Model file for the job. Use its own axes, mm. A direction names the side the tool comes from. Coordinates: 2 decimals unless noted, no trailing zeros. Write each loop counter-clockwise with the first axis right and the second up, starting at its lowest first coordinate (ties: lowest second). Pieces come first, ordered by that corner, then holes. Notation, with made-up numbers: (11, 78.25) -> (43, 78.25) arc R31 cw to (43, 110.25) -> close; hole circle Ø10 at (-3.75, -18). An arc over 180 degrees is marked (long way). Answer as a JSON object with one key per item and string values. Group by question number.
from build123d import *

# Parameters (mm, degrees)
F1_DEPTH  = 5.715
F2_R      = 1.143
F3_DEPTH  = 3.175
F5_R      = 4.445
F6_DEPTH  = 19.05
F4_R      = 3.175
F7_DEPTH  = 19.05
F8_R      = 4.7625
F9_DEPTH  = 6.35
F10_R     = 1.143
F11_DEPTH = 6.35
F13_DEPTH = 3.175
F14_R     = 3.175
F15_DEPTH = 0.396875


with BuildPart() as f1:
    # F0 (on Top) → F1 (new body)
    with BuildSketch(Plane.XY):
        with BuildLine():
            ThreePointArc((-9.989334, -1.5875), (-15.875, -6.096), (-21.760666, -1.5875))
            Line((-21.760666, -1.5875), (-36.5252, -1.5875))
            Line((-36.5252, -1.5875), (-36.5252, -20.6375))
            Line((-36.5252, -20.6375), (25.4, -20.6375))
            Line((25.4, -20.6375), (25.4, -1.5875))
            Line((25.4, -1.5875), (21.760666, -1.5875))
            ThreePointArc((21.760666, -1.5875), (15.875, -6.096), (9.989334, -1.5875))
            Line((9.989334, -1.5875), (-9.989334, -1.5875))
        make_face()
    extrude(amount=F1_DEPTH)

    # F2 (on face) → F3 (join)
    with BuildSketch(Plane.XZ.offset(20.6375)):
        with BuildLine():
            ThreePointArc((-25.53469, 45.96899), (-27.779754, 45.039054), (-28.70969, 42.79399))
            Line((-28.70969, 42.79399), (-28.70969, 5.715))
            Line((-28.70969, 5.715), (-23.289328, 5.715))
            Line((-23.289328, 5.715), (-23.289328, 40.549224))
            Line((-23.289328, 40.549224), (12.156438, 40.549224))
            Line((12.156438, 40.549224), (12.156438, 5.715))
            Line((12.156438, 5.715), (17.5768, 5.715))
            Line((17.5768, 5.715), (17.5768, 42.79399))
            ThreePointArc((17.5768, 42.79399), (16.646864, 45.039054), (14.4018, 45.96899))
            Line((14.4018, 45.96899), (-25.53469, 45.96899))
        make_face()
        with Locations((-25.53469, 42.79399)):
            Circle(F2_R, mode=Mode.SUBTRACT)
        with Locations((14.4018, 2.8575)):
            Circle(F2_R)
    extrude(amount=-F3_DEPTH)

    # F5 (on face) → F6 (join, through all)
    with BuildSketch(Plane.XZ.offset(20.6375)):
        with Locations((-29.142933, 2.8575)):
            Circle(F5_R)
        with Locations((0, 2.8575)):
            Circle(F5_R)
    extrude(amount=-F6_DEPTH)

    # F4 (on face) → F7 (cut, through all)
    with BuildSketch(Plane.XZ.offset(20.6375)):
        with Locations((-29.142933, 2.8575)):
            Circle(F4_R)
        with Locations((0, 2.8575)):
            Circle(F4_R)
    extrude(amount=-F7_DEPTH, mode=Mode.SUBTRACT)

    # F8 (on face) → F9 (cut)
    with BuildSketch(Plane.XZ.offset(20.6375)):
        with Locations((-29.142933, 2.8575)):
            Circle(F8_R)
        with Locations((0, 2.8575)):
            Circle(F8_R)
    extrude(amount=-F9_DEPTH, mode=Mode.SUBTRACT)

    # F10 (on face) → F11 (cut)
    with BuildSketch(Plane.XZ.offset(20.6375)):
        with Locations((14.4018, 2.8575)):
            Circle(F10_R)
    extrude(amount=-F11_DEPTH, mode=Mode.SUBTRACT)

    # F12 (on face) → F13 (join, through all)
    with BuildSketch(Plane.XZ.offset(20.6375)):
        with BuildLine():
            Line((-25.332933, 0), (-19.724361, 0))
            ThreePointArc((-19.724361, 0), (-21.110093, 8.545056), (-28.70969, 12.69046))
            Line((-28.70969, 12.69046), (-28.70969, 7.600253))
            ThreePointArc((-28.70969, 7.600253), (-24.790664, 4.791192), (-25.332933, 0))
        make_face()
    extrude(amount=-F13_DEPTH)

    # F14 (on face) → F15 (join)
    with BuildSketch(Plane.XZ.offset(14.2875)):
        with Locations((0, 2.8575)):
            Circle(F14_R)
        with Locations((-29.142933, 2.8575)):
            Circle(F14_R)
    extrude(amount=-F15_DEPTH)


solid = f1.part
(1) Cut at A-A on x = -7. List the corners of the cut face in (y, z) (1 decimal).
(2) Wall check: probe 1 along Z at (x, y) = (-18, -19.25) (3 decimals); probe 2 along Z at (x, y) = (0, -6.5); probe 3 along Z at (x, y) = (17.5, -15) (3 decimals). Give the ranges that are in metal, low to high.
(3) Cut at B-B on z = 32.5. List the corners of the cut face in (x, y).
(4) Cut at C-C on y = -8.25. Give the number of separate pieces and of enclosed holes in the cut face, plus the area to 3 significant figures.
(5) 3-axis set-ups, long thin cutter, end or side, ignore diameter. For faces 1 (the face through (-35, -11, 5.715)), 2 (the face through (-15, -11, 0)), 3 (the face through (15.492, -17.507, 3.201)), 4 (the face through (-6, -19, 40.549)), 5 (the face through (-7, -17.462, 41)): which of +Z, -Z, +X, -X, +Y, -Y reach the whole face in a straight line?
(6) Pull direction X, two halves, no side cores. Call faces 6 (the face through (14, -11, 0)), 7 (the face through (0, -14.288, 3)), 8 (the face through (-27.755, -19.072, 45.064)): released by +X, released by -X, zero draft, split by the parting line, or undercut.
(7) Pin check, flat tips, straight feed: pin 1 (1.6 mm diameter, centred on y = -19.5, z = 33.5, fed in from -X); pin 2 (10 mm diameter, centred on x = -15.5, y = -11, fed in from -Z); pin 3 (1.8 mm diameter, centred on x = 14.4, z = 2.86, fed in from +Y). Stop position of each tip, or through.
(8) Cut at D-D on x = 0. List the corners of the cut face in (y, z), plus the area to 3 significant figures.
Results found:
{
 "1": {"outline": "(-20.6, 0) -> (-1.6, 0) -> (-1.6, 5.7) -> (-20.6, 5.7) -> close; (-20.6, 40.5) -> (-17.5, 40.5) -> (-17.5, 46) -> (-20.6, 46) -> close"},
 "2": {"probe 1": "z = 0 to 5.715, 40.549 to 45.969", "probe 2": "z = -1.59 to -0.32, 6.03 to 7.3", "probe 3": "z = 0 to 5.715"},
 "3": {"outline": "(-28.71, -20.64) -> (-23.29, -20.64) -> (-23.29, -17.46) -> (-28.71, -17.46) -> close; (12.16, -20.64) -> (17.58, -20.64) -> (17.58, -17.46) -> (12.16, -17.46) -> close"},
 "4": {"separate pieces": "1", "enclosed holes": "2", "area": "321 mm²"},
 "5": {"face 1": "+Z, -X, +Y, -Y", "face 2": "-Z, +Y, -Y", "face 3": "-Y", "face 4": "+Y, -Y", "face 5": "+Z, +X, -X, +Y"},
 "6": {"face 6": "zero draft", "face 7": "undercut", "face 8": "released by -X"},
 "7": {"pin 1": "stops at x = -28.71", "pin 2": "stops at z = 0", "pin 3": "stops at y = -5.61"},
 "8": {"outline": "(-20.64, 40.55) -> (-17.46, 40.55) -> (-17.46, 45.97) -> (-20.64, 45.97) -> close; (-14.29, -1.59) -> (-1.59, -1.59) -> (-1.59, -0.32) -> (-13.89, -0.32) -> (-13.89, 6.03) -> (-1.59, 6.03) -> (-1.59, 7.3) -> (-14.29, 7.3) -> close", "area": "52.0 mm²"}
}
